```python
from build123d import *

# Parameters (mm, degrees)
SKETCH1_R                = 2.75
SKETCH1_R_2              = 2.25
BOSS_EXTRUDE1_DEPTH      = 4
SKETCH3_W                = 10
SKETCH3_H                = 42
BOSS_EXTRUDE3_DEPTH      = 15
SKETCH4_R                = 2.5
CUT_EXTRUDE1_DEPTH       = 58.280013966
CHAMFER1_SIZE            = 0.75
BOSS_EXTRUDE5_DEPTH      = 30
BOSS_EXTRUDE5_DEPTH_BACK = 70
SKETCH8_W                = 15
SKETCH8_H                = 10
SKETCH10_W               = 10
SKETCH10_H               = 3
CUT_EXTRUDE4_DEPTH       = 113.942463228
BOSS_EXTRUDE6_START      = 23
SKETCH11_W               = 10
SKETCH11_H               = 19
SKETCH11_R               = 2.5
BOSS_EXTRUDE6_DEPTH      = 23
BOSS_EXTRUDE7_DEPTH      = 3
BOSS_EXTRUDE8_DEPTH      = 10
BOSS_EXTRUDE9_DEPTH      = 10
CHAMFER2_SIZE            = 5
CHAMFER3_SIZE            = 10
CHAMFER4_SIZE            = 5
BOSS_EXTRUDE10_REACH     = 112.603


with BuildPart() as part:
    # Sketch1 → Boss-Extrude1 (new body)
    with BuildSketch(Plane(origin=(0, 0, 0), x_dir=(1, 0, 0), z_dir=(0, 1, 0))):
        Polygon((-34, 0), (-34, 40), (34, 40), (34, 0), (34, -2), (-34, -2), align=None)
        with Locations(Location((-19, 22.5, 0), (0, 0, 270))):
            Circle(SKETCH1_R, mode=Mode.SUBTRACT)
        with Locations(Location((19, 22.5, 0), (0, 0, 270))):
            Circle(SKETCH1_R, mode=Mode.SUBTRACT)
        with Locations(Location((-14, 15, 0), (0, 0, 270))):
            Circle(SKETCH1_R_2, mode=Mode.SUBTRACT)
        with Locations(Location((14, 15, 0), (0, 0, 270))):
            Circle(SKETCH1_R_2, mode=Mode.SUBTRACT)
        with Locations(Location((0, 6, 0), (0, 0, 270))):
            Circle(SKETCH1_R, mode=Mode.SUBTRACT)
    extrude(amount=BOSS_EXTRUDE1_DEPTH)

    # Sketch3 → Boss-Extrude3 (add)
    with BuildSketch(Plane(origin=(0, 4, 0), x_dir=(1, 0, 0), z_dir=(0, 1, 0))):
        with Locations((-29, 19)):
            Rectangle(SKETCH3_W, SKETCH3_H)
        with Locations((29, 19)):
            Rectangle(SKETCH3_W, SKETCH3_H)
    extrude(amount=BOSS_EXTRUDE3_DEPTH)

    # Sketch4 → Cut-Extrude1 (cut, through all)
    with BuildSketch(Plane(origin=(0, 0, -40), x_dir=(-1, 0, 0), z_dir=(0, 0, -1))):
        with Locations((-29, 11)):
            Circle(SKETCH4_R)
        with Locations((29, 11)):
            Circle(SKETCH4_R)
    extrude(amount=-CUT_EXTRUDE1_DEPTH, mode=Mode.SUBTRACT)

    # Chamfer1
    chamfer1_edges = [part.edges().sort_by_distance(p)[0] for p in [
        (-19, 4, -25.25),
        (19, 4, -25.25),
        (0, 4, -8.75),
    ]]
    chamfer(chamfer1_edges, length=CHAMFER1_SIZE)

    # Sketch8 → Boss-Extrude5 (add, two sides: drawn at the far end of the back side and taken through both)
    with BuildSketch(Plane.XZ.offset(-BOSS_EXTRUDE5_DEPTH_BACK)):
        with Locations((26.5, 7)):
            Rectangle(SKETCH8_W, SKETCH8_H)
    extrude(amount=BOSS_EXTRUDE5_DEPTH + BOSS_EXTRUDE5_DEPTH_BACK)

    # Sketch10 → Cut-Extrude4 (cut, through all)
    with BuildSketch(Plane(origin=(0, 70, 0), x_dir=(1, 0, 0), z_dir=(0, 1, 0))):
        with Locations((26.5, -7)):
            Rectangle(SKETCH10_W, SKETCH10_H)
    extrude(amount=-CUT_EXTRUDE4_DEPTH, mode=Mode.SUBTRACT)

    # Sketch11 → Boss-Extrude6 (add)
    # profile 1 of 2: a face of its own
    with BuildSketch(Plane(origin=(0, 0, -40), x_dir=(-1, 0, 0), z_dir=(0, 0, -1)).offset(BOSS_EXTRUDE6_START)):
        with Locations((-29, 9.5)):
            Rectangle(SKETCH11_W, SKETCH11_H)
        with Locations((-29, 11)):
            Circle(SKETCH11_R, mode=Mode.SUBTRACT)
    # profile 2 of 2: a face of its own
    with BuildSketch(Plane(origin=(0, 0, -40), x_dir=(-1, 0, 0), z_dir=(0, 0, -1)).offset(BOSS_EXTRUDE6_START)):
        with Locations((29, 9.5)):
            Rectangle(SKETCH11_W, SKETCH11_H)
        with Locations((29, 11)):
            Circle(SKETCH11_R, mode=Mode.SUBTRACT)
    extrude(amount=-BOSS_EXTRUDE6_DEPTH)

    # Sketch12 → Boss-Extrude7 (add)
    with BuildSketch(Plane(origin=(0, 0, -40), x_dir=(-1, 0, 0), z_dir=(0, 0, -1))):
        Polygon((-24, 0), (-24, 4), (24, 4), (24, 0), (34, 0), (34, -20), (-34, -20), (-34, 0), align=None)
    extrude(amount=BOSS_EXTRUDE7_DEPTH)

    # Sketch13 → Boss-Extrude8 (add)
    with BuildSketch(Plane.ZY.offset(34)):
        Polygon((-63, 0), (-43, -20), (-43, 0), align=None)
    extrude(amount=-BOSS_EXTRUDE8_DEPTH)

    # Sketch14 → Boss-Extrude9 (add)
    with BuildSketch(Plane(origin=(34, 0, 0), x_dir=(0, 0, -1), z_dir=(1, 0, 0))):
        Polygon((43, 0), (43, -20), (63, 0), align=None)
    extrude(amount=-BOSS_EXTRUDE9_DEPTH)

    # Chamfer2
    chamfer2_edges = [part.edges().sort_by_distance(p)[0] for p in [
        (24, 11.5, 2),
    ]]
    chamfer(chamfer2_edges, length=CHAMFER2_SIZE - 0.0001)  # a hair under: the kernel refuses the full size

    # Chamfer3
    chamfer3_edges = [part.edges().sort_by_distance(p)[0] for p in [
        (19, 2, 2),
    ]]
    chamfer(chamfer3_edges, length=CHAMFER3_SIZE - 0.0001)  # a hair under: the kernel refuses the full size

    # Chamfer4
    chamfer4_edges = [part.edges().sort_by_distance(p)[0] for p in [
        (26.50005, 19, 2),
    ]]
    chamfer(chamfer4_edges, length=CHAMFER4_SIZE)

    # Sketch15 → Boss-Extrude10 (add, up to next)
    with BuildSketch(Plane.ZY.offset(-24), mode=Mode.PRIVATE) as boss_extrude10_sk1:
        Polygon((-43, -20), (-43, 4), (-63, 4), (-63, 0), align=None)
    boss_extrude10_tool1 = extrude(boss_extrude10_sk1.sketch, amount=BOSS_EXTRUDE10_REACH, mode=Mode.PRIVATE) - part.part
    add(boss_extrude10_tool1.solids().sort_by_distance((24, -4.190476, -50.619048))[0])


solid = part.part
```
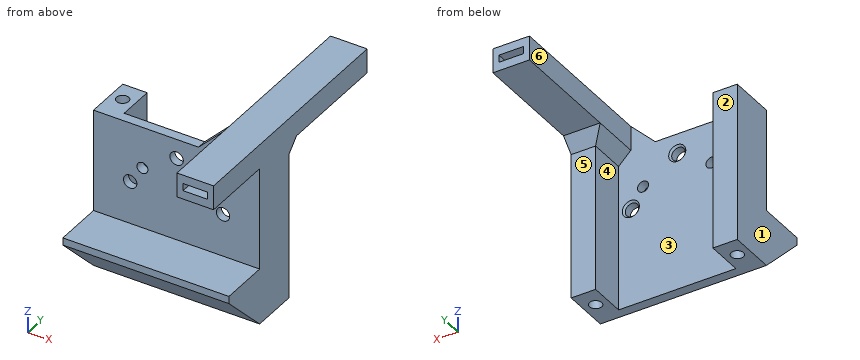
The model under review builds one solid part; all positions refer to its coordinate system, in mm. Face numbers are marked on the shaded views. A direction names the side the tool comes from. Round coordinates to 2 decimals unless told otherwise and drop trailing zeros. Loops run counter-clockwise (first coordinate to the right, second up) from the corner with the lowest first, then second, coordinate; pieces in that order, holes last. Notation, with made-up numbers: (12, 19) - (17, 19) arc R11 ccw to (17, 38) - close; hole circle Ø8 at (-33.5, 6.25). An arc over 180 degrees is marked (long way). Write each question's results on one line, items separated by ' | '. Start each with the question number.
Q1. Draft analysis for pull direction X (two halves, no side actions). For the marked faces 1, 2 and 3, state which applies: pulls with the +X half, pulls with the -X half, needs draft (parallel to the pull), parting line crosses it, or undercut.
Q2. Wall thickness on line 1 along X through (y, z) = (1, -15); line 2 along Z through (x, y) = (29.5, 24.5); line 3 along Y through (x, z) = (-29, -36.5): over which ranges is each line inside the solid? List them lowest first. Write a range as [from, to].
Q3. Take a section at B-B on x = 29. Give the boundary of the cut face in (y, z), plus the area to 3 significant figures.
Q4. Take a section at D-D on z = -6. Give the boundary of the cut face in (x, y), plus the area to 3 significant figures.
Q5. Take a section at C-C on z = -15. Give the boundary of the cut face in (x, y), plus the area to 3 significant figures.
Q6. Insertion check: P1, Ø10, axis at x = 7, y = -13.5, coming from the +Z side; P2, Ø3, axis at x = -26.5, z = -35.5, coming from the +Y side; P3, Ø5, axis at x = 0, z = -6, coming from the +Y side; P4, Ø10, axis at x = 12.5, z = -2.5, coming from the -Y side. Each pin has a flat end and moves straight along its axis. Give the tip position at first contact, or say it passes through.
Q7. Take a section at A-A on y = 11. Give the number of separate pieces and of enclosed holes in the cut face, plus the area to 4 significant figures.
Q8. Tool access review of the marked faces 4, 5 and 6: name each direction out of +Z, -Z, +X, -X, +Y, -Y from which nothing blocks a thin tool from reaching the whole face with its end or side.
Data:
1) face 1: pulls with the -X half | face 2: needs draft | face 3: undercut
2) line 1: x = [-34, -16.25], [-11.75, 11.75], [16.25, 34] | line 2: z = [2, 5.5], [8.5, 12] | line 3: y = [0, 8.5], [13.5, 19]
3) outline: (-30, 2) - (0, 2) - (0, -40) - (-20, -40) - (-20, -43) - (0, -63) - (8.5, -63) - (8.5, 2) - (13.5, 2) - (13.5, -63) - (19, -63) - (19, -3) - (24, 2) - (70, 2) - (70, 5.5) - (-30, 5.5) - close; (-30, 8.5) - (70, 8.5) - (70, 12) - (-30, 12) - close | area: 1,880 mm²
4) outline: (-34, 0) - (-2.75, 0) - (-2.75, 3.25) - (-3.5, 4) - (-24, 4) - (-24, 19) - (-34, 19) - close; (2.75, 0) - (34, 0) - (34, 19) - (24, 19) - (24, 4) - (3.5, 4) - (2.75, 3.25) - close; hole circle Ø5 at (-29, 11); hole circle Ø5 at (29, 11) | area: 510 mm²
5) outline: (-34, 0) - (-16.25, 0) - (-16.25, 4) - (-24, 4) - (-24, 19) - (-34, 19) - close; (-11.75, 0) - (11.75, 0) - (11.75, 4) - (-11.75, 4) - close; (16.25, 0) - (34, 0) - (34, 19) - (24, 19) - (24, 4) - (16.25, 4) - close; hole circle Ø5 at (-29, 11); hole circle Ø5 at (29, 11) | area: 497 mm²
6) P1: stops at z = -40 | P2: stops at y = 19 | P3: passes through | P4: stops at y = 0
7) separate pieces: 3 | enclosed holes: 1 | area: 782.5 mm²
8) face 4: -Z, +Y | face 5: -Z, +X, -X, +Y | face 6: +Z, -Z, -X, +Y
